```python
from build123d import *

# Parameters (mm, degrees)
F0_W     = 114.3
F0_H     = 63.5
F1_DEPTH = 76.2
F2_R     = 50.8
F3_DEPTH = 50.8
F4_R     = 6.35
F5_DEPTH = 76.2
F6_R     = 25.4
F7_DEPTH = 87.376


with BuildPart() as f1:
    # F0 (on Front) → F1 (new body)
    with BuildSketch(Plane.XZ):
        Rectangle(F0_W, F0_H)
    extrude(amount=F1_DEPTH)

    # F2 (on face) → F3 (cut)
    with BuildSketch(Plane(origin=(-57.15, 0, 0), x_dir=(0, -1, 0), z_dir=(-1, 0, 0))):
        with Locations((76.2, 31.75)):
            Circle(F2_R)
    extrude(amount=-F3_DEPTH, mode=Mode.SUBTRACT)

    # F4 (on face) → F5 (cut)
    with BuildSketch(Plane.XZ.offset(76.2)):
        with Locations((21.054188, 6.35)):
            Circle(F4_R)
    extrude(amount=-F5_DEPTH, mode=Mode.SUBTRACT)

    # F6 (on face) → F7 (cut)
    with BuildSketch(Plane.XY.offset(31.75)):
        with Locations((57.15, -38.1)):
            Circle(F6_R)
    extrude(amount=-F7_DEPTH, mode=Mode.SUBTRACT)


solid = f1.part
```
CAD build for the part. Positions are in the model's coordinates, mm. A direction names the side the tool comes from. Round coordinates to 2 decimals unless told otherwise and drop trailing zeros. Loops run counter-clockwise (first coordinate to the right, second up) from the corner with the lowest first, then second, coordinate; pieces in that order, holes last. Notation, with made-up numbers: (-22.75, 59) - (-10.75, 59) arc R26 cw to (-10.75, 84) - close; hole circle Ø4 at (68.25, 37.25). An arc over 180 degrees is marked (long way). Return JSON: item names as keys, results as strings. Group by question number.
Q1. Band-saw the part on B-B on z = 6.35. Give the cut face in (x, y), plus the area to 3 significant figures.
Q2. Two-plate mould, pull along X, no slides. Class faces 1 (the face through (57.15, -70, 0)), 2 (the face through (-6.35, -56, 12)), 3 (the face through (24.468, -38.633, 11.704)), 4 (the face through (12, -29, 31.75)): +X half, -X half, draft (parallel to the pull), parting line (faces both ways), or undercut.
Q3. Band-saw the part on A-A on x = 40. Give the cut face in (y, z).
Q4. Band-saw the part on D-D on z = -4.5. Give the cut face in (x, y).
Q5. Flat gauge pins, fed straight in: pin 1 Ø4 at (x, z) = (-5, 13.5) entering from +Y; pin 2 Ø3 at (y, z) = (-63, -12.5) entering from -X; pin 3 Ø5 at (x, z) = (-18.5, -5.5) entering from -Y. Where does each tip first touch, or does it go through?
Q6. Drill centre lines: line 1 along Y through (x, z) = (41.5, 3); line 2 along X through (y, z) = (-25.5, 7); line 3 along Z through (x, y) = (20, -48.5). Where is each one in solid material? Low to high. Write a range as [from, to].
Q7. Tool access for faces 5 (the face through (-32.106, -39.886, -3.774)), 6 (the face through (57.15, -6, 0)): list every direction of +Z, -Z, +X, -X, +Y, -Y with a clear straight run to the whole face (end or side of a thin tool).
Q8. Band-saw the part on C-C on y = -36. Give the cut face in (x, z), plus the area to 3 significant figures.
Solutions:
{
 "1": {"outline": "(-57.15, -32.21) - (-6.35, -32.21) - (-6.35, -76.2) - (14.7, -76.2) - (14.7, 0) - (-57.15, 0) - close; (27.4, -76.2) - (57.15, -76.2) - (57.15, -63.5) arc R25.4 cw to (57.15, -12.7) - (57.15, 0) - (27.4, 0) - close", "area": "4,490 mm^2"},
 "2": {"face 1": "+X half", "face 2": "-X half", "face 3": "undercut", "face 4": "draft"},
 "3": {"outline": "(-76.2, -31.75) - (-56.84, -31.75) - (-56.84, 31.75) - (-76.2, 31.75) - close; (-19.36, -31.75) - (0, -31.75) - (0, 31.75) - (-19.36, 31.75) - close"},
 "4": {"outline": "(-57.15, -40.61) - (-6.35, -40.61) - (-6.35, -76.2) - (57.15, -76.2) - (57.15, -63.5) arc R25.4 cw to (57.15, -12.7) - (57.15, 0) - (-57.15, 0) - close"},
 "5": {"pin 1": "stops at y = 0", "pin 2": "stops at x = -6.35", "pin 3": "stops at y = -44.57"},
 "6": {"line 1": "y = [-76.2, -58.11], [-18.09, 0]", "line 2": "x = [-57.15, 14.74], [27.37, 35.1]", "line 3": "z = [-31.75, 0.09], [12.61, 31.75]"},
 "7": {"face 5": "+Z, -X, -Y", "face 6": "+Z, -Z, +X, +Y, -Y"},
 "8": {"outline": "(-57.15, -31.75) - (31.84, -31.75) - (31.84, 31.75) - (-6.35, 31.75) - (-6.35, 0.69) - (-57.15, 0.69) - close; hole circle Ø12.7 at (21.05, 6.35)", "area": "3,950 mm^2"}
}
